The figure shows three views and two pictorial views of one solid part (mm, origin at its lowest corner). Answer the questions. A direction names the side the tool comes from. Round coordinates to 2 decimals unless told otherwise and drop trailing zeros. Write each loop counter-clockwise with the first axis right and the second up, starting at its lowest first coordinate (ties: lowest second). Pieces come first, ordered by that corner, then holes. Notation, with made-up numbers: (3.5, 58) -> (17.5, 58) arc R18 ccw to (17.5, 87) -> close; hole circle Ø8 at (-34.75, 26.25). An arc over 180 degrees is marked (long way). One line per item, written item: value.
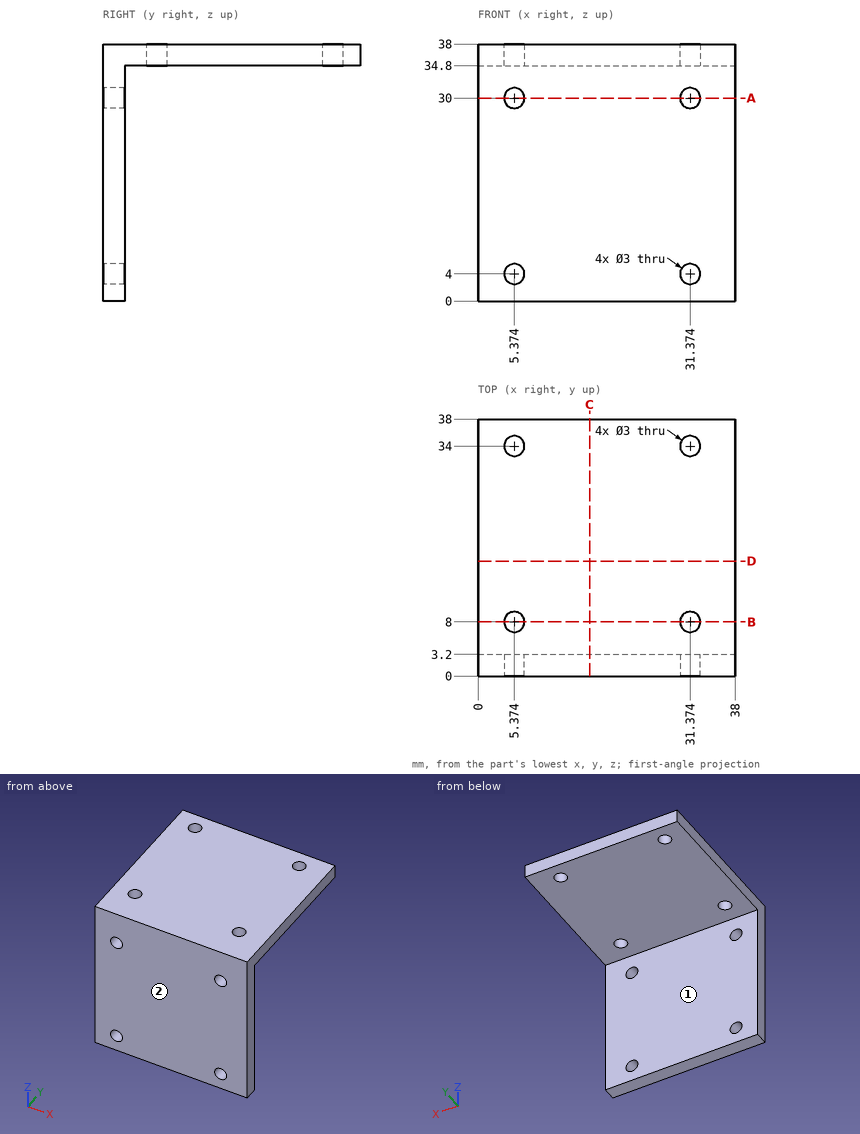
(1) Find section D-D on y = 17. Give the vertices of the cut face in (x, z).
Reported:
outline: (0, 34.8) -> (38, 34.8) -> (38, 38) -> (0, 38) -> close
(2) A tool of negligible diameter and unlimited length cuts with its end or side. For the marked faces 1 and 2, from which of +Z, -Z, +X, -X, +Y, -Y can it reach the whole face along a straight path? Write none if from no direction.
Reported:
face 1: -Z, +X, -X, +Y
face 2: +Z, -Z, +X, -X, -Y
(3) Find section B-B on y = 8. Give the vertices of the cut face in (x, z) (1 decimal).
Reported:
outline: (0, 34.8) -> (3.9, 34.8) -> (3.9, 38) -> (0, 38) -> close; (6.9, 34.8) -> (29.9, 34.8) -> (29.9, 38) -> (6.9, 38) -> close; (32.9, 34.8) -> (38, 34.8) -> (38, 38) -> (32.9, 38) -> close
(4) Find section C-C on x = 16.5. Give the vertices of the cut face in (y, z), plus the area to 3 significant figures.
Reported:
outline: (0, 0) -> (3.2, 0) -> (3.2, 34.8) -> (38, 34.8) -> (38, 38) -> (0, 38) -> close
area: 233 mm2
(5) Find section A-A on z = 30. Give the vertices of the cut face in (x, y) (1 decimal), plus the area to 3 significant figures.
Reported:
outline: (0, 0) -> (3.9, 0) -> (3.9, 3.2) -> (0, 3.2) -> close; (6.9, 0) -> (29.9, 0) -> (29.9, 3.2) -> (6.9, 3.2) -> close; (32.9, 0) -> (38, 0) -> (38, 3.2) -> (32.9, 3.2) -> close
area: 102 mm2
(6) Consider probe 1 along Y at (x, z) = (15, 6); probe 2 along Z at (x, y) = (5, 13.5). Determine where each line is inside the solid, lowest interval first.
Reported:
probe 1: y = 0 to 3.2
probe 2: z = 34.8 to 38
(7) Flat-ended cylindrical pins translate along their axes: pin 1 Ø12 at (x, y) = (13, 22.5) entering from -Z; pin 2 Ø3.5 at (x, z) = (31.37, 30) entering from +Y. Find the tip coordinate at first contact, or state that the pin passes through.
Reported:
pin 1: stops at z = 34.8
pin 2: stops at y = 3.2
